from build123d import *

# Parameters (mm, degrees)
SKETCH3_R          = 4.087752765
CUT_EXTRUDE1_DEPTH = 3.5


with BuildPart() as part:
    # Sketch1 → 5.63 mm bottom to pen tip (revolve)
    with BuildSketch(Plane.XY):
        Polygon((0, 0), (3, 0), (3.2, 5.5), (5.5, 5.5), (5.75, 8.5), (5.75, 22.3), (7, 22.3), (8.25, 22.55), (8.25, 24.05), (7, 24.3), (5.75, 24.3), (5.75, 37.3), (0, 37.3), align=None)
    revolve(axis=Axis((0, -143.950460456, 0), (0, 1, 0)))

    # Sketch2 → Cut-Revolve1 (revolve, cut)
    with BuildSketch(Plane(origin=(0, 0, 0), x_dir=(0, 0, -1), z_dir=(1, 0, 0))):
        Polygon((0.75, -5.63), (0.75, -0.43), (2.575, -0.43), (2.575, 6.87), (5, 6.87), (5, 39.162156903), (0, 39.162156903), (0, -5.63), align=None)
    revolve(axis=Axis((0, -1000, 0), (0, 1, 0)), mode=Mode.SUBTRACT)

    # Sketch3 → Cut-Extrude1 (cut)
    with BuildSketch(Plane(origin=(0, 0, 0), x_dir=(-1, 0, 0), z_dir=(0, -1, 0))):
        Circle(SKETCH3_R)
    extrude(amount=-CUT_EXTRUDE1_DEPTH, mode=Mode.SUBTRACT)


solid = part.part
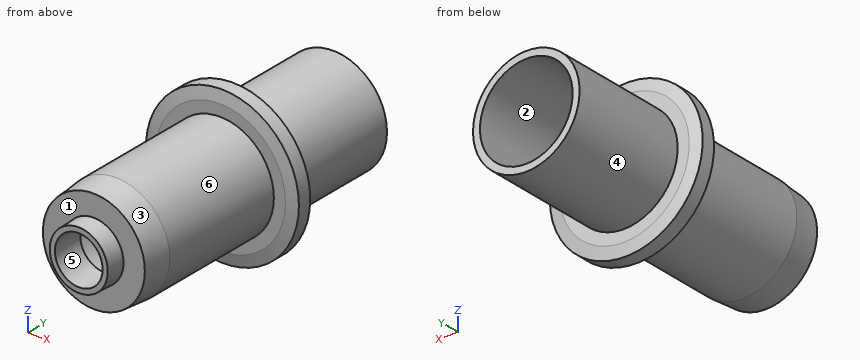
Source: CAD feature listing. Evaluate the final solid. Frame: model axes, mm. Face numbers are marked on the shaded views. A direction names the side the tool comes from. Round coordinates to 2 decimals unless told otherwise and drop trailing zeros. Loops run counter-clockwise (first coordinate to the right, second up) from the corner with the lowest first, then second, coordinate; pieces in that order, holes last.
Q1. Access query for the marked faces 4, 5 and 6. Directions: +Z, -Z, +X, -X, +Y, -Y. A direction counts if a zero-diameter tool reaches every point of the face in a straight line with its end or side. Return the directions, or none.
Q2. First-contact query: P1, Ø7, axis at x = -2.5, z = 3.5, coming from the -Y side; P2, Ø3, axis at x = 0, y = 31, coming from the +Z side; P3, Ø4, axis at x = 0, z = 0, coming from the -Y side; P4, Ø4, axis at y = 17, z = 6.5, coming from the +X side. Flat tips, straight axial feed; report the tip coordinate or a pass-through.
Q3. Mould query, pull axis Z, two halves, no side actions, for the marked faces 1, 2 and 3. Classes: pulls with the +Z half, pulls with the -Z half, needs draft (parallel to the pull), parting line crosses it, or undercut.
Q4. Section C-C, the plane y = 13. Return loops of the section in (x, z), plus the area to 3 significant figures.
Q5. Ray query, line 1 (X direction, y = 30, z = 0); line 2 (X direction, y = 5.4, z = 0) (3 decimals). Return the intervals inside material, ascending.
Solutions:
1. face 4: +Y
1. face 5: +Y, -Y
1. face 6: -Y
2. P1: stops at y = 3.5
2. P2: stops at z = 5.75
2. P3: passes through
2. P4: stops at x = 3.58
3. face 1: needs draft
3. face 2: undercut
3. face 3: parting line crosses it
4. outline: circle Ø11.5 at (0, 0); hole circle Ø10 at (0, 0)
4. area: 25.3 mm2
5. line 1: x = -5.75 to -5, 5 to 5.75
5. line 2: x = -3.196 to -2.575, 2.575 to 3.196
